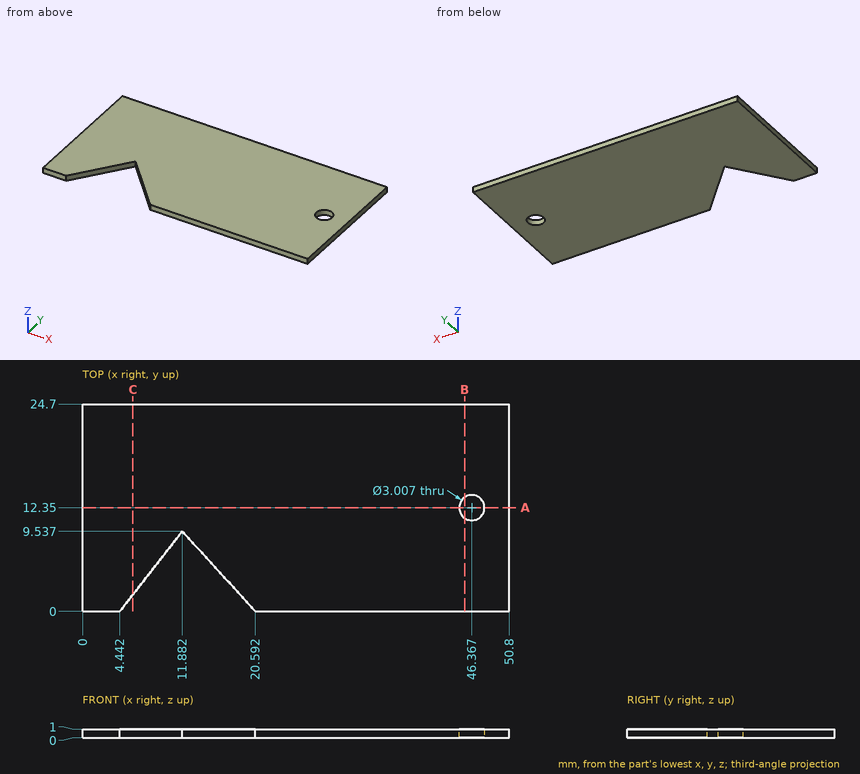
Geometry check sheet. Reference: drawing and pictorial views, mm from the part's lowest x, y, z. Give positions to 0.01 mm unless a question says otherwise; leave off trailing zeros. Order: outer loops, then holes, each group sorted by start corner. A loop starts at its lowest first (then second) coordinate and runs counter-clockwise, first axis right, second up. Notation, with made-up numbers: M -27,-33.75 L -18,-33.75 A24 ccw -18,-12.75 Z; hole C -33,-14.75 d4. An arc over 180 degrees is marked long. Answer as CSV lines item,"result". Start each with the question number.
Item 1: Cross-section at B-B on x = 45.5. Enter the section's corners in (y, z).
Item 2: Cross-section at C-C on x = 6. Enter the section's corners in (y, z).
Item 3: Cross-section at A-A on y = 12.35. Enter the section's corners in (x, z).
Item 4: Thickness scan on line 1 (X direction, y = 3.5, z = 0.15) (1 decimal); line 2 (Y direction, x = 17, z = 0.5) (1 decimal); line 3 (X direction, y = 6.5, z = 0.55) (1 decimal). Record the ranges inside material, lowest first. Write a range as [from, to].
Established:
1,outline,"M 0,0 L 11.12,0 L 11.12,1 L 0,1 Z; M 13.58,0 L 24.7,0 L 24.7,1 L 13.58,1 Z"
2,outline,"M 2,0 L 24.7,0 L 24.7,1 L 2,1 Z"
3,outline,"M 0,0 L 44.86,0 L 44.86,1 L 0,1 Z; M 47.87,0 L 50.8,0 L 50.8,1 L 47.87,1 Z"
4,line 1,"x = [0, 7.2], [17.4, 50.8]"
4,line 2,"y = [3.9, 24.7]"
4,line 3,"x = [0, 9.5], [14.7, 50.8]"
